Here's how the part is built. I have some questions about the finished solid (model axes, mm). A direction names the side the tool comes from. Coordinates: 2 decimals unless noted, no trailing zeros. Order: outer loops, then holes, each group sorted by start corner. A loop starts at its lowest first (then second) coordinate and runs counter-clockwise, first axis right, second up. Notation, with made-up numbers: (67, 83.25) - (81, 83.25) arc R29 cw to (81, 120.25) - close; hole circle Ø10 at (3, -15.5). An arc over 180 degrees is marked (long way). Answer in a Markdown table with one row per item. Add a question column.
Item 1: If I drill on line 1 along X through (y, z) = (222, -11); line 2 along Y through (x, z) = (-633, -14.5); line 3 along Y through (x, z) = (637, 1), over which ranges is the centre line in solid material (lowest first)? Write a range as from..to.
Item 2: Will these pins go through, and if not, where does the flat tip stop? pin 1 Ø4 at (y, z) = (104, -6) entering from -X; pin 2 Ø4 at (x, z) = (-17.5, -6.5) entering from -Y; pin 3 Ø7 at (y, z) = (281, 4) entering from +X.
Item 3: I want a section at B-B (z = 0). Please give me the cut outline in (x, y), plus the area to 3 significant figures.
Item 4: On a 3-axis mill with a long thin cutter (end or side, diameter ignored), from which of +Z, -Z, +X, -X, +Y, -Y can I reach the whole of each face in a straight line? I mean faces 4 (the cylindrical face through (10.36, -18.59, 2.44)), 5 (the flat face through (-412, 190, -11.798)), 6 (the flat face through (740, 0, 0)), 7 (the flat face through (412, 195, 11.798)), 8 (the cylindrical face through (411.81, 374.75, -0.18)). Say none if no direction works.
Item 5: I want a section at C-C (x = -507). Please give me the cut outline in (y, z), plus the area to 3 significant figures.
Item 6: Thinking about a two-plate mould opening in X: for faces 1 (the flat face through (384.425, 192, 0)), 2 (the flat face through (-740, 0, 0)), 3 (the cylindrical face through (-411.81, 374.75, -0.18)), which applies, +X half, -X half, draft (parallel to the pull), parting line (faces both ways), or undercut?
Item 7: I want a section at A-A (y = 42.5). Please give me the cut outline in (x, z).
```python
from build123d import *

# Parameters (mm, degrees)
SKETCH1_W           = 1480
SKETCH1_H           = 18.75
BOSS_EXTRUDE2_START = -438.446590399
BOSS_EXTRUDE2_DEPTH = 54.021923435


# Read off the part's stored shape, not the designer's step: Boss-Extrude2
with BuildPart() as part:
    # Sketch1 → Revolve1 (revolve)
    with BuildSketch(Plane(origin=(0, 0, 0), x_dir=(1, 0, 0), z_dir=(0, 1, 0))):
        with Locations((0, 9.375)):
            Rectangle(SKETCH1_W, SKETCH1_H)
    revolve(axis=Axis((270.12195122, 0, 0), (-1, 0, 0)))

    # Boss-Extrude2 outline → Boss-Extrude2 (add)
    with BuildSketch(Plane.YZ.offset(BOSS_EXTRUDE2_START)):
        with BuildLine():
            Line((14.573043819, -11.797834286), (370.573043819, -11.797834286))
            ThreePointArc((370.573043819, -11.797834286), (374.75, 0), (370.573043819, 11.797834286))
            Line((370.573043819, 11.797834286), (14.573043819, 11.797834286))
            ThreePointArc((14.573043819, 11.797834286), (18.75, 0), (14.573043819, -11.797834286))
        make_face()
    boss_extrude2 = extrude(amount=BOSS_EXTRUDE2_DEPTH)

    # Mirror1: Boss-Extrude2 across plane
    add(boss_extrude2.mirror(Plane(origin=(0, 0, 0), x_dir=(0, 0, 1), z_dir=(1, 0, 0))))


solid = part.part
```
Values follow:
| question | item | result |
|---|---|---|
| 1 | line 1 | x = -438.45..-384.42, 384.42..438.45 |
| 1 | line 2 | y = -11.89..11.89 |
| 1 | line 3 | y = -18.72..18.72 |
| 2 | pin 1 | stops at x = -438.45 |
| 2 | pin 2 | stops at y = -18.2 |
| 2 | pin 3 | stops at x = 438.45 |
| 3 | outline | (-740, -18.75) - (740, -18.75) - (740, 18.75) - (438.45, 18.75) - (438.45, 374.75) - (384.42, 374.75) - (384.42, 18.75) - (-384.42, 18.75) - (-384.42, 374.75) - (-438.45, 374.75) - (-438.45, 18.75) - (-740, 18.75) - close |
| 3 | area | 94,000 mm^2 |
| 4 | face 4 | none |
| 4 | face 5 | -Z, +X, -X, +Y |
| 4 | face 6 | +Z, -Z, +X, +Y, -Y |
| 4 | face 7 | +Z, +X, -X, +Y |
| 4 | face 8 | +X, -X, +Y |
| 5 | outline | circle Ø37.5 at (0, 0) |
| 5 | area | 1,100 mm^2 |
| 6 | face 1 | undercut |
| 6 | face 2 | -X half |
| 6 | face 3 | draft |
| 7 | outline | (-438.45, -11.8) - (-384.42, -11.8) - (-384.42, 11.8) - (-438.45, 11.8) - close; (384.42, -11.8) - (438.45, -11.8) - (438.45, 11.8) - (384.42, 11.8) - close |
